```python
from build123d import *

# Parameters (mm, degrees)
TAPERFILLET_R                     = 3.175
HOLEPATTERN_COUNT                 = 16
POCKETFILLETS_R                   = 6.35
PIPE_TAP_DRILL_FOR_1_2_TAP1_D     = 17.8562
PIPE_TAP_DRILL_FOR_1_2_TAP1_DEPTH = 46.99
PIPE_TAP_DRILL_FOR_1_2_TAP1_TIP   = 5.364543693


with BuildPart() as part:
    # Sketch1 → Revolve1 (revolve)
    with BuildSketch(Plane.XY):
        Polygon((0, -15.24), (0, 0), (-58.4454, 0), (-58.4454, -12.7), (-54.1274, -12.7), (-54.1274, -21.971), (-58.4454, -21.971), (-58.4454, -31.75), (-48.9331, -31.75), (-48.9331, -15.24), align=None)
        Polygon((-58.4454, 0), (0, 0), (0, 15.24), (-43.6499, 15.24), (-43.6499, 54.0385), (-49.9999, 54.0385), (-49.9999, 44.5262), (-58.236420675, 44.5262), (-58.4454, 31.8262), (-58.4454, 21.971), (-54.1274, 21.971), (-54.1274, 12.7), (-58.4454, 12.7), align=None)
    revolve(axis=Axis((0, 31.75, 0), (0, -1, 0)))

    # TaperFillet
    taperfillet_edges = [part.edges().sort_by_distance(p)[0] for p in [
        (58.236420675, 44.5262, 0),
    ]]
    fillet(taperfillet_edges, radius=TAPERFILLET_R)

    # Sketch4 → Tap Drill for 1/4-28 Tap1 (revolve, cut)
    with BuildSketch(Plane(origin=(0, 0, -58.4454), x_dir=(0, 1, 0), z_dir=(1, 0, 0))):
        Polygon((0, 0), (0, 20.675388061), (2.7051, 19.05), (2.7051, 0), align=None)
    tap_drill_for_1_4_28_tap1 = revolve(axis=Axis((0, 0, -64.7954), (0, 0, 1)), mode=Mode.SUBTRACT)

    # HolePattern: Tap Drill for 1/4-28 Tap1 ×16 about axis
    holepattern_axis = Axis((0, -12.7, 0), (0, 1, 0))
    for i in range(1, HOLEPATTERN_COUNT):
        add(tap_drill_for_1_4_28_tap1.rotate(holepattern_axis, i * 360 / HOLEPATTERN_COUNT), mode=Mode.SUBTRACT)

    # PocketFillets
    pocketfillets_edges = [part.edges().sort_by_distance(p)[0] for p in [
        (43.6499, 15.24, 0),
        (48.9331, -15.24, 0),
    ]]
    fillet(pocketfillets_edges, radius=POCKETFILLETS_R)

    # Pipe Tap Drill for 1/2 Tap1
    with Locations(Plane(origin=(0, 15.24, 0), x_dir=(1, 0, 0), z_dir=(0, 1, 0))):
        with Locations((0, 0)):
            Hole(PIPE_TAP_DRILL_FOR_1_2_TAP1_D / 2, depth=PIPE_TAP_DRILL_FOR_1_2_TAP1_DEPTH)
            with Locations((0, 0, -(PIPE_TAP_DRILL_FOR_1_2_TAP1_DEPTH + PIPE_TAP_DRILL_FOR_1_2_TAP1_TIP / 2))):  # 118° drill point
                Cone(0, PIPE_TAP_DRILL_FOR_1_2_TAP1_D / 2, PIPE_TAP_DRILL_FOR_1_2_TAP1_TIP, mode=Mode.SUBTRACT)


solid = part.part
```
Check sheet for the modelled part. Datum: model origin and axes. Units: mm. A direction names the side the tool comes from. Coordinates: 2 decimals unless noted, no trailing zeros. Loops run counter-clockwise (first coordinate to the right, second up) from the corner with the lowest first, then second, coordinate; pieces in that order, holes last.
1) Release check for a two-part mould opening along X. For faces 4 (the face through (12, 44.526, 49)), 5 (the face through (-16.7, 1.5, 46.2)), 6 (the face through (46.38, -0.178, 35.563)) record: released by +X, released by -X, zero draft, split by the parting line, or undercut.
2) Access from +Z, -Z, +X, -X, +Y, -Y to the whole of each face (thin tool, end or side, straight path). Record for faces 1 (the face through (-8.516, -0.213, -2.682)), 2 (the face through (52, 12.7, 17)), 3 (the face through (49.054, -2.147, 1.646)).
3) Gauge pin test, flat ends, axial feed: pin 1 (1.5 mm diameter, centred on x = 43, y = 14, fed in from -Z); pin 2 (5 mm diameter, centred on y = -16.5, z = 39, fed in from +X); pin 3 (12 mm diameter, centred on x = 3, z = -15.5, fed in from -Y); pin 4 (16 mm diameter, centred on x = 0, z = 0, fed in from -Y). Record the tip position at first contact, or that the pin passes through.
4) Sectioned sample at A-A (y = -4.5). Record the boundary of the cut face in (x, z).
5) Sectioned sample at B-B (z = 32). Count the separate pieces of the cut face and the enclosed holes in it, and give its area (3 significant figures).
6) Sectioned sample at D-D (y = 39). Record the boundary of the cut face in (x, z).
7) Material ranges on probe 1 along X at (y, z) = (45, -0.5); probe 2 along Z at (x, y) = (46, 0); probe 3 along X at (y, z) = (-25.75, 0), recorded low to high.
Check sheet entries:
1. face 4: zero draft
1. face 5: undercut
1. face 6: split by the parting line
2. face 1: +Y, -Y
2. face 2: none
2. face 3: +X
3. pin 1: stops at z = -33.83
3. pin 2: stops at x = 39.97
3. pin 3: stops at y = -15.24
3. pin 4: passes through
4. outline: circle Ø116.89 at (0, 0); hole circle Ø17.86 at (0, 0)
5. separate pieces: 1
5. enclosed holes: 2
5. area: 4,450 mm2
6. outline: circle Ø116.65 at (0, 0); hole circle Ø87.3 at (0, 0)
7. probe 1: x = -50 to -43.65, 43.65 to 50
7. probe 2: z = -36.05 to -21.98, -16.13 to -2.71, 2.71 to 16.13, 21.98 to 36.05
7. probe 3: x = -58.45 to -48.93, 48.93 to 58.45
